Can you work these out from the model? Positions are in its coordinate system, mm. Face numbers are marked on the shaded views. A direction names the side the tool comes from. Give positions to 0.01 mm unless a question says otherwise; leave off trailing zeros. Order: outer loops, then holes, each group sorted by start corner. A loop starts at its lowest first (then second) coordinate and runs counter-clockwise, first axis right, second up. Notation, with made-up numbers: (-27.5, 45) -> (-18.5, 45) arc R22 ccw to (-18.5, 69) -> close; hole circle Ø1 at (21.25, 73.25). An arc over 180 degrees is marked (long way). Answer as a JSON object with one key per item and string values.
```python
from build123d import *

# Parameters (mm, degrees)
SKETCH1_W           = 457.2
SKETCH1_H           = 228.6
BOSS_EXTRUDE1_DEPTH = 609.6
SHELL2_T            = -12.7
CUT_EXTRUDE2_REACH  = 772.525
CUT_EXTRUDE3_REACH  = 692.02
SKETCH4_W           = 31.75
SKETCH4_H           = 34.29
SKETCH4_W_2         = 36.83
SKETCH4_H_2         = 11.43
CUT_EXTRUDE17_DEPTH = 55.88


with BuildPart() as part:
    # Sketch1 → Boss-Extrude1 (new body)
    with BuildSketch(Plane(origin=(0, 0, 0), x_dir=(1, 0, 0), z_dir=(0, 1, 0))):
        Rectangle(SKETCH1_W, SKETCH1_H)
    extrude(amount=BOSS_EXTRUDE1_DEPTH)

    # Shell2
    shell2_openings = [part.faces().sort_by_distance(p)[0] for p in [
        (0, 609.6, 0),
    ]]
    offset(amount=SHELL2_T, openings=shell2_openings, kind=Kind.INTERSECTION)

    # Sketch3 → Cut-Extrude2 (cut, up to next)
    with BuildSketch(Plane(origin=(228.6, 0, 0), x_dir=(0, 0, -1), z_dir=(1, 0, 0)), mode=Mode.PRIVATE) as cut_extrude2_sk1:
        with BuildLine():
            Line((-25.4, 76.2), (-25.4, 533.4))
            ThreePointArc((-25.4, 533.4), (0, 558.8), (25.4, 533.4))
            Line((25.4, 533.4), (25.4, 76.2))
            ThreePointArc((25.4, 76.2), (0, 50.8), (-25.4, 76.2))
        make_face()
    cut_extrude2_tool1 = extrude(cut_extrude2_sk1.sketch, amount=-CUT_EXTRUDE2_REACH, mode=Mode.PRIVATE) & part.part
    add(cut_extrude2_tool1.solids().sort_by_distance((228.6, 304.8, 0))[0], mode=Mode.SUBTRACT)

    # Sketch4 → Cut-Extrude3 (cut, up to next)
    with BuildSketch(Plane(origin=(0, 0, -114.3), x_dir=(-1, 0, 0), z_dir=(0, 0, -1)), mode=Mode.PRIVATE) as cut_extrude3_sk1:
        with Locations((109.44862115, 351.970372474)):
            Rectangle(SKETCH4_W, SKETCH4_H)
    cut_extrude3_tool1 = extrude(cut_extrude3_sk1.sketch, amount=-CUT_EXTRUDE3_REACH, mode=Mode.PRIVATE) & part.part
    # Sketch4 → Cut-Extrude3 (cut, up to next)
    with BuildSketch(Plane(origin=(0, 0, -114.3), x_dir=(-1, 0, 0), z_dir=(0, 0, -1)), mode=Mode.PRIVATE) as cut_extrude3_sk2:
        with Locations((109.44862115, 317.680372474)):
            Rectangle(SKETCH4_W, SKETCH4_H)
    cut_extrude3_tool2 = extrude(cut_extrude3_sk2.sketch, amount=-CUT_EXTRUDE3_REACH, mode=Mode.PRIVATE) & part.part
    # Sketch4 → Cut-Extrude3 (cut, up to next)
    with BuildSketch(Plane(origin=(0, 0, -114.3), x_dir=(-1, 0, 0), z_dir=(0, 0, -1)), mode=Mode.PRIVATE) as cut_extrude3_sk3:
        with Locations((141.19862115, 317.680372474)):
            Rectangle(SKETCH4_W, SKETCH4_H)
    cut_extrude3_tool3 = extrude(cut_extrude3_sk3.sketch, amount=-CUT_EXTRUDE3_REACH, mode=Mode.PRIVATE) & part.part
    # Sketch4 → Cut-Extrude3 (cut, up to next)
    with BuildSketch(Plane(origin=(0, 0, -114.3), x_dir=(-1, 0, 0), z_dir=(0, 0, -1)), mode=Mode.PRIVATE) as cut_extrude3_sk4:
        with Locations((141.19862115, 351.970372474)):
            Rectangle(SKETCH4_W, SKETCH4_H)
    cut_extrude3_tool4 = extrude(cut_extrude3_sk4.sketch, amount=-CUT_EXTRUDE3_REACH, mode=Mode.PRIVATE) & part.part
    # Sketch4 → Cut-Extrude3 (cut, up to next)
    with BuildSketch(Plane(origin=(0, 0, -114.3), x_dir=(-1, 0, 0), z_dir=(0, 0, -1)), mode=Mode.PRIVATE) as cut_extrude3_sk5:
        with Locations((138.56658474, 419.56196337)):
            Rectangle(SKETCH4_W_2, SKETCH4_H_2)
    cut_extrude3_tool5 = extrude(cut_extrude3_sk5.sketch, amount=-CUT_EXTRUDE3_REACH, mode=Mode.PRIVATE) & part.part
    # Sketch4 → Cut-Extrude3 (cut, up to next)
    with BuildSketch(Plane(origin=(0, 0, -114.3), x_dir=(-1, 0, 0), z_dir=(0, 0, -1)), mode=Mode.PRIVATE) as cut_extrude3_sk6:
        with Locations((138.56658474, 408.13196337)):
            Rectangle(SKETCH4_W_2, SKETCH4_H_2)
    cut_extrude3_tool6 = extrude(cut_extrude3_sk6.sketch, amount=-CUT_EXTRUDE3_REACH, mode=Mode.PRIVATE) & part.part
    # Sketch4 → Cut-Extrude3 (cut, up to next)
    with BuildSketch(Plane(origin=(0, 0, -114.3), x_dir=(-1, 0, 0), z_dir=(0, 0, -1)), mode=Mode.PRIVATE) as cut_extrude3_sk7:
        with Locations((101.73658474, 419.56196337)):
            Rectangle(SKETCH4_W_2, SKETCH4_H_2)
    cut_extrude3_tool7 = extrude(cut_extrude3_sk7.sketch, amount=-CUT_EXTRUDE3_REACH, mode=Mode.PRIVATE) & part.part
    # Sketch4 → Cut-Extrude3 (cut, up to next)
    with BuildSketch(Plane(origin=(0, 0, -114.3), x_dir=(-1, 0, 0), z_dir=(0, 0, -1)), mode=Mode.PRIVATE) as cut_extrude3_sk8:
        with Locations((101.73658474, 408.13196337)):
            Rectangle(SKETCH4_W_2, SKETCH4_H_2)
    cut_extrude3_tool8 = extrude(cut_extrude3_sk8.sketch, amount=-CUT_EXTRUDE3_REACH, mode=Mode.PRIVATE) & part.part
    add(cut_extrude3_tool1.solids().sort_by_distance((-109.448621, 351.970372, -114.3))[0], mode=Mode.SUBTRACT)
    add(cut_extrude3_tool2.solids().sort_by_distance((-109.448621, 317.680372, -114.3))[0], mode=Mode.SUBTRACT)
    add(cut_extrude3_tool3.solids().sort_by_distance((-141.198621, 317.680372, -114.3))[0], mode=Mode.SUBTRACT)
    add(cut_extrude3_tool4.solids().sort_by_distance((-141.198621, 351.970372, -114.3))[0], mode=Mode.SUBTRACT)
    add(cut_extrude3_tool5.solids().sort_by_distance((-138.566585, 419.561963, -114.3))[0], mode=Mode.SUBTRACT)
    add(cut_extrude3_tool6.solids().sort_by_distance((-138.566585, 408.131963, -114.3))[0], mode=Mode.SUBTRACT)
    add(cut_extrude3_tool7.solids().sort_by_distance((-101.736585, 419.561963, -114.3))[0], mode=Mode.SUBTRACT)
    add(cut_extrude3_tool8.solids().sort_by_distance((-101.736585, 408.131963, -114.3))[0], mode=Mode.SUBTRACT)

    # Sketch11 → Cut-Extrude17 (cut)
    with BuildSketch(Plane.ZY.offset(228.6)):
        with BuildLine():
            Line((-65.38521106, 17.765922532), (-88.113220021, 17.765922532))
            ThreePointArc((-88.113220021, 17.765922532), (-94.463220021, 24.115922532), (-88.113220021, 30.465922532))
            Line((-88.113220021, 30.465922532), (-65.38521106, 30.465922532))
            ThreePointArc((-65.38521106, 30.465922532), (-59.03521106, 24.115922532), (-65.38521106, 17.765922532))
        make_face()
    extrude(amount=-CUT_EXTRUDE17_DEPTH, mode=Mode.SUBTRACT)


solid = part.part
```
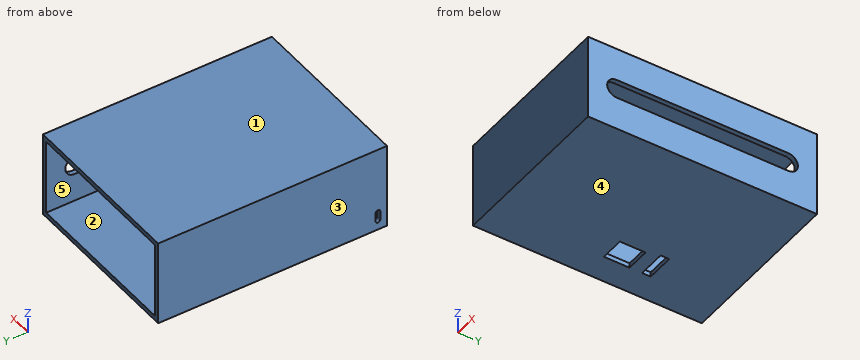
1. If we section it at D-D on y = 511: Please give me the cut outline in (x, z).
Worked answers:
{"outline": "(-228.6, -114.3) -> (228.6, -114.3) -> (228.6, -25.4) -> (215.9, -25.4) -> (215.9, -101.6) -> (-215.9, -101.6) -> (-215.9, 101.6) -> (215.9, 101.6) -> (215.9, 25.4) -> (228.6, 25.4) -> (228.6, 114.3) -> (-228.6, 114.3) -> close"}
2. Please list where these lines run through material, in increasing order: L1, parallel to Z at x = -136, y = 225; L2, parallel to X at y = 191.5, z = 91.5; L3, parallel to Y at x = 96, z = -74.5.
Worked answers:
{"L1": "-114.3 to -101.6, 101.6 to 114.3", "L2": "-228.6 to -215.9, 215.9 to 228.6", "L3": "0 to 12.7"}
3. For the marked faces 4 and 5, which set-ups out of +Z, -Z, +X, -X, +Y, -Y let a thin tool reach every point of the face, with its end or its side?
Worked answers:
{"face 4": "-Z, +X, -X, +Y, -Y", "face 5": "+Y"}
4. If we section it at A-A on x = -113.5: Please give me the cut outline in (y, z), then the cut area to 3 significant figures.
Worked answers:
{"outline": "(0, -114.3) -> (300.54, -114.3) -> (300.54, -101.6) -> (12.7, -101.6) -> (12.7, 101.6) -> (609.6, 101.6) -> (609.6, 114.3) -> (0, 114.3) -> close; (369.12, -114.3) -> (402.42, -114.3) -> (402.42, -101.6) -> (369.12, -101.6) -> close; (425.28, -114.3) -> (609.6, -114.3) -> (609.6, -101.6) -> (425.28, -101.6) -> close", "area": "16,900 mm²"}
5. If we section it at C-C on z = 0: Please give me the cut outline in (x, y).
Worked answers:
{"outline": "(-228.6, 0) -> (228.6, 0) -> (228.6, 50.8) -> (215.9, 50.8) -> (215.9, 12.7) -> (-215.9, 12.7) -> (-215.9, 609.6) -> (-228.6, 609.6) -> close; (215.9, 558.8) -> (228.6, 558.8) -> (228.6, 609.6) -> (215.9, 609.6) -> close"}
6. If we mould it in two halves opening along X, with no side actions, what happens to the marked faces 1, 2 and 3? For each: +X half, -X half, draft (parallel to the pull), parting line (faces both ways), or undercut.
Worked answers:
{"face 1": "draft", "face 2": "undercut", "face 3": "-X half"}
7. If we section it at B-B on y = 347.5: Please give me the cut outline in (x, z), then the cut area to 3 significant figures.
Worked answers:
{"outline": "(-228.6, -114.3) -> (-157.07, -114.3) -> (-157.07, -101.6) -> (-215.9, -101.6) -> (-215.9, 101.6) -> (215.9, 101.6) -> (215.9, 25.4) -> (228.6, 25.4) -> (228.6, 114.3) -> (-228.6, 114.3) -> close; (-93.57, -114.3) -> (228.6, -114.3) -> (228.6, -25.4) -> (215.9, -25.4) -> (215.9, -101.6) -> (-93.57, -101.6) -> close", "area": "15,300 mm²"}
8. Will these pins go through, and if not, where does the flat tip stop? pin 1 Ø3 at (x, z) = (-125.5, -18) entering from +Y; pin 2 Ø14 at (x, z) = (-112, -109) entering from -Y.
Worked answers:
{"pin 1": "y = 12.7", "pin 2": "y = 0"}
